from build123d import *

# Parameters (mm, degrees)
CROQUIS1_W              = 12
CROQUIS1_H              = 19
CROQUIS1_W_2            = 8
CROQUIS1_H_2            = 15
SALIENTE_EXTRUIR1_DEPTH = 186.5
CROQUIS2_W              = 12
CROQUIS2_H              = 15
CORTAR_EXTRUIR1_DEPTH   = 12
CROQUIS3_R              = 2.5
CORTAR_EXTRUIR2_DEPTH   = 19
SKETCH1_W               = 186.5
SKETCH1_H               = 19
CUT_EXTRUDE1_DEPTH      = 13
SKETCH2_W               = 7
SKETCH2_H               = 19
BOSS_EXTRUDE1_DEPTH     = 10
SKETCH3_R               = 2.5
CUT_EXTRUDE2_DEPTH      = 10
FILLET1_R               = 5
FILLET2_R               = 5


with BuildPart() as part:
    # Croquis1 → Saliente-Extruir1 (new body, symmetric)
    with BuildSketch(Plane(origin=(0, 0, 0), x_dir=(0, 0, -1), z_dir=(1, 0, 0))):
        Rectangle(CROQUIS1_W, CROQUIS1_H)
        Rectangle(CROQUIS1_W_2, CROQUIS1_H_2, mode=Mode.SUBTRACT)
    extrude(amount=SALIENTE_EXTRUIR1_DEPTH, both=True)

    # Croquis2 → Cortar-Extruir1 (cut)
    with BuildSketch(Plane.XY.offset(6)):
        with Locations((-180.5, 0)):
            Rectangle(CROQUIS2_W, CROQUIS2_H)
        with Locations((180.5, 0)):
            Rectangle(CROQUIS2_W, CROQUIS2_H)
    extrude(amount=-CORTAR_EXTRUIR1_DEPTH, mode=Mode.SUBTRACT)

    # Croquis3 → Cortar-Extruir2 (cut)
    with BuildSketch(Plane(origin=(0, 9.5, 0), x_dir=(1, 0, 0), z_dir=(0, 1, 0))):
        with Locations((-180.5, 0)):
            Circle(CROQUIS3_R)
        with Locations((180.5, 0)):
            Circle(CROQUIS3_R)
    extrude(amount=-CORTAR_EXTRUIR2_DEPTH, mode=Mode.SUBTRACT)

    # Sketch1 → Cut-Extrude1 (cut, through all)
    with BuildSketch(Plane.XY.offset(6)):
        with Locations((93.25, 0)):
            Rectangle(SKETCH1_W, SKETCH1_H)
    extrude(amount=-CUT_EXTRUDE1_DEPTH, mode=Mode.SUBTRACT)

    # Sketch2 → Boss-Extrude1 (add)
    with BuildSketch(Plane.XY.offset(6)):
        with Locations((-3.5, 0)):
            Rectangle(SKETCH2_W, SKETCH2_H)
    boss_extrude1 = extrude(amount=BOSS_EXTRUDE1_DEPTH)

    # Sketch3 → Cut-Extrude2 (cut)
    with BuildSketch(Plane(origin=(0, 0, 0), x_dir=(0, 0, -1), z_dir=(1, 0, 0))):
        with Locations((-11, 0)):
            Circle(SKETCH3_R)
    cut_extrude2 = extrude(amount=-CUT_EXTRUDE2_DEPTH, mode=Mode.SUBTRACT)

    # Fillet1
    fillet1_edges = [part.edges().sort_by_distance(p)[0] for p in [
        (-3.5, 9.5, 16),
        (-3.5, -9.5, 16),
    ]]
    fillet(fillet1_edges, radius=FILLET1_R)

    # Mirror1: Boss-Extrude1, Cut-Extrude2 across plane
    add(boss_extrude1.mirror(Plane.XY))
    add(cut_extrude2.mirror(Plane.XY), mode=Mode.SUBTRACT)

    # Fillet2
    fillet2_edges = [part.edges().sort_by_distance(p)[0] for p in [
        (-3.5, -9.5, -16),
        (-3.5, 9.5, -16),
    ]]
    fillet(fillet2_edges, radius=FILLET2_R)


solid = part.part
Read the model definition and answer for the solid it produces. Units are mm, in the model's axes. A direction names the side the tool comes from. Round coordinates to 2 decimals unless told otherwise and drop trailing zeros. Write each loop counter-clockwise with the first axis right and the second up, starting at its lowest first coordinate (ties: lowest second). Pieces come first, ordered by that corner, then holes. Notation, with made-up numbers: (-19.75, 55) - (4.25, 55) arc R31 ccw to (4.25, 83) - close; hole circle Ø2 at (32, 87.5). An arc over 180 degrees is marked (long way). Use a Markdown table: item, result.
(1) The part is cut by section C-C (z = 0). Write down the section's boundary in (x, y).
Reported:
| item | result |
|---|---|
| outline | (-186.5, -9.5) - (-183, -9.5) - (-183, -7.5) - (-186.5, -7.5) - close; (-186.5, 7.5) - (-183, 7.5) - (-183, 9.5) - (-186.5, 9.5) - close; (-178, -9.5) - (0, -9.5) - (0, -7.5) - (-178, -7.5) - close; (-178, 7.5) - (0, 7.5) - (0, 9.5) - (-178, 9.5) - close |
(2) The part is cut by section A-A (y = 0). Write down the section's boundary in (x, z), then the cut area to 3 significant figures.
Reported:
| item | result |
|---|---|
| outline | (-174.5, -6) - (-7, -6) - (-7, -8.5) - (0, -8.5) - (0, -4) - (-174.5, -4) - close; (-174.5, 4) - (0, 4) - (0, 8.5) - (-7, 8.5) - (-7, 6) - (-174.5, 6) - close; (-7, -16) - (0, -16) - (0, -13.5) - (-7, -13.5) - close; (-7, 13.5) - (0, 13.5) - (0, 16) - (-7, 16) - close |
| area | 768 mm2 |
(3) The part is cut by section D-D (x = -83.5). Write down the section's boundary in (y, z), then the cut area to 3 significant figures.
Reported:
| item | result |
|---|---|
| outline | (-9.5, -6) - (9.5, -6) - (9.5, 6) - (-9.5, 6) - close; hole (-7.5, -4) - (7.5, -4) - (7.5, 4) - (-7.5, 4) - close |
| area | 108 mm2 |
(4) The mould has two halves that part along X. Classify faces 4 (the cylindrical face through (-178.115, -8.486, -0.751)), 5 (the flat face through (-86, 0, -4)), 6 (the flat face through (-7, -2, 9)): released by +X, released by -X, zero draft, split by the parting line, or undercut.
Reported:
| item | result |
|---|---|
| face 4 | undercut |
| face 5 | zero draft |
| face 6 | released by -X |
(5) Which of the six approach directions +Z, -Z, +X, -X, +Y, -Y give full straight-line access (tool end or side, diameter ignored) to faces 1 (the flat face through (-95, 0, 6)), 2 (the cylindrical face through (-3.45, 8, 14.57)), 3 (the flat face through (-7, -2, -9))?
Reported:
| item | result |
|---|---|
| face 1 | +Z, -X, +Y, -Y |
| face 2 | +Z, +X, -X, +Y |
| face 3 | -Z, -X, +Y, -Y |
(6) The part is cut by section B-B (x = -180.5). Write down the section's boundary in (y, z), then the cut area to 3 significant figures.
Reported:
| item | result |
|---|---|
| outline | (-9.5, -6) - (-7.5, -6) - (-7.5, -2.5) - (-9.5, -2.5) - close; (-9.5, 2.5) - (-7.5, 2.5) - (-7.5, 6) - (-9.5, 6) - close; (7.5, -6) - (9.5, -6) - (9.5, -2.5) - (7.5, -2.5) - close; (7.5, 2.5) - (9.5, 2.5) - (9.5, 6) - (7.5, 6) - close |
| area | 28.0 mm2 |
(7) Each of these flat-tipped pins is pushed along its axis until it touches: pin 1 Ø3 at (x, y) = (-126.5, 1) entering from -Z; pin 2 Ø11 at (y, z) = (0.5, -8.5) entering from -X; pin 3 Ø4 at (x, y) = (-109, 5) entering from +Z. Where does it stop, or does it pass through?
Reported:
| item | result |
|---|---|
| pin 1 | z = -6 |
| pin 2 | x = -174.5 |
| pin 3 | z = 6 |
(8) Straight lines are drawn through the part: line 1 along X through (y, z) = (-8.85, 0); line 2 along Z through (x, y) = (-124.5, -5); line 3 along Z through (x, y) = (-180.5, -8.15). For each, find the intervals that lie inside material, in ascending order. Write a range as [from, to].
Reported:
| item | result |
|---|---|
| line 1 | [-186.5, -183], [-178, 0] |
| line 2 | [-6, -4], [4, 6] |
| line 3 | [-6, -2.5], [2.5, 6] |
